Build history of the part. All positions in model axes, mm. A direction names the side the tool comes from. Give positions to 0.01 mm unless a question says otherwise; leave off trailing zeros. Order: outer loops, then holes, each group sorted by start corner. A loop starts at its lowest first (then second) coordinate and runs counter-clockwise, first axis right, second up. Notation, with made-up numbers: (-34.5, 27) - (6.5, 27) arc R10 cw to (6.5, 41) - close; hole circle Ø2 at (-31.5, -18.5). An arc over 180 degrees is marked (long way). Answer in a Markdown table with one row per item.
```python
from build123d import *

# Parameters (mm, degrees)
ESBO_O1_R                = 1.6
ESBO_O1_W                = 21
ESBO_O1_H                = 42
RESSALTO_EXTRUS_O1_DEPTH = 3
FILETE1_R                = 7


with BuildPart() as part:
    # Esboço1 → Ressalto-extrusão1 (new body)
    with BuildSketch(Plane.XY):
        with BuildLine():
            Line((-14.5, 27.75), (-14.5, -27.75))
            Line((-14.5, -27.75), (-2.5, -27.75))
            ThreePointArc((-2.5, -27.75), (0, -25.25), (2.5, -27.75))
            Line((2.5, -27.75), (14.5, -27.75))
            Line((14.5, -27.75), (14.5, 27.75))
            Line((14.5, 27.75), (2.5, 27.75))
            ThreePointArc((2.5, 27.75), (0, 25.25), (-2.5, 27.75))
            Line((-2.5, 27.75), (-14.5, 27.75))
        make_face()
        with Locations((-5, -24.75)):
            Circle(ESBO_O1_R, mode=Mode.SUBTRACT)
        with Locations((5, -24.75)):
            Circle(ESBO_O1_R, mode=Mode.SUBTRACT)
        Rectangle(ESBO_O1_W, ESBO_O1_H, mode=Mode.SUBTRACT)
        with Locations((-5, 24.75)):
            Circle(ESBO_O1_R, mode=Mode.SUBTRACT)
        with Locations((5, 24.75)):
            Circle(ESBO_O1_R, mode=Mode.SUBTRACT)
    extrude(amount=RESSALTO_EXTRUS_O1_DEPTH)

    # Filete1
    filete1_edges = [part.edges().sort_by_distance(p)[0] for p in [
        (-14.5, -27.75, 1.5),
        (-14.5, 27.75, 1.5),
        (-2.5, 27.75, 1.5),
        (2.5, 27.75, 1.5),
        (14.5, 27.75, 1.5),
        (14.5, -27.75, 1.5),
        (2.5, -27.75, 1.5),
        (-2.5, -27.75, 1.5),
    ]]
    fillet(filete1_edges, radius=FILETE1_R)


solid = part.part
```
1. Cut at B-B on x = -5. Write the cut outline in (y, z).
Check result:
| item | result |
|---|---|
| outline | (-27.6, 0) - (-26.35, 0) - (-26.35, 3) - (-27.6, 3) - close; (-23.15, 0) - (-21, 0) - (-21, 3) - (-23.15, 3) - close; (21, 0) - (23.15, 0) - (23.15, 3) - (21, 3) - close; (26.35, 0) - (27.6, 0) - (27.6, 3) - (26.35, 3) - close |
2. Probe line 1 (X direction, y = -5, z = 1.2); line 2 (Y direction, x = -5, z = 2.3); line 3 (Y direction, x = -5.5, z = 0.35). List the from-to ranges inside material, lowest first.
Check result:
| item | result |
|---|---|
| line 1 | x = -14.5 to -10.5, 10.5 to 14.5 |
| line 2 | y = -27.6 to -26.35, -23.15 to -21, 21 to 23.15, 26.35 to 27.6 |
| line 3 | y = -27.69 to -26.27, -23.23 to -21, 21 to 23.23, 26.27 to 27.69 |
3. Two-plate mould, pull along X, no slides. Class faces 3 (the face through (-3.917, -27.286, 1.521)), 4 (the face through (-12.5, 25.65, 1.52)), 5 (the face through (11, 0, 3)), 6 (the face through (12.4, -25.75, 1.52)): +X half, -X half, draft (parallel to the pull), parting line (faces both ways), or undercut.
Check result:
| item | result |
|---|---|
| face 3 | undercut |
| face 4 | -X half |
| face 5 | draft |
| face 6 | +X half |
4. Drop flat-ended pins along their axis: P1, Ø1.9, axis at x = -5, y = 24.75, coming from the -Z side; P2, Ø1, axis at x = -0.5, z = 2.5, coming from the +Y side. Give the stop position or say it passes through.
Check result:
| item | result |
|---|---|
| P1 | passes through |
| P2 | stops at y = 25.46 |
5. Cut at D-D on y = -24. Write the cut outline in (x, z), and give its area (3 significant figures).
Check result:
| item | result |
|---|---|
| outline | (-13.7, 0) - (-6.41, 0) - (-6.41, 3) - (-13.7, 3) - close; (-3.59, 0) - (3.59, 0) - (3.59, 3) - (-3.59, 3) - close; (6.41, 0) - (13.7, 0) - (13.7, 3) - (6.41, 3) - close |
| area | 65.2 mm² |
6. Cut at C-C on x = 8.75. Write the cut outline in (y, z).
Check result:
| item | result |
|---|---|
| outline | (-27.64, 0) - (-21, 0) - (-21, 3) - (-27.64, 3) - close; (21, 0) - (27.64, 0) - (27.64, 3) - (21, 3) - close |
7. Which spindle directions (+Z, -Z, +X, -X, +Y, -Y) get a long thin tool onto all of the face, cutting with end or side? Do faces 1 (the face through (-7, -27.75, 1)), 2 (the face through (0, -21, 1)). Say none if no direction does.
Check result:
| item | result |
|---|---|
| face 1 | +Z, -Z, +X, -X, -Y |
| face 2 | +Z, -Z |
8. Cut at A-A on y = -15.5. Write the cut outline in (x, z).
Check result:
| item | result |
|---|---|
| outline | (-14.5, 0) - (-10.5, 0) - (-10.5, 3) - (-14.5, 3) - close; (10.5, 0) - (14.5, 0) - (14.5, 3) - (10.5, 3) - close |
